from build123d import *

# Parameters (mm, degrees)
SKETCH_1_R          = 13.5
EXTRUDE_1_DEPTH     = 2
SKETCH_2_R          = 6.5
EXTRUDE_2_DEPTH     = 13
SKETCH_3_R          = 4
CUT_EXTRUDE_1_DEPTH = 15
SKETCH_4_R          = 1.5
CUT_EXTRUDE_2_DEPTH = 15


with BuildPart() as part:
    # 草图1 → 凸台-拉伸1 (new body)
    with BuildSketch(Plane.XY):
        Circle(SKETCH_1_R)
    extrude(amount=EXTRUDE_1_DEPTH)

    # 草图2 → 凸台-拉伸2 (add)
    with BuildSketch(Plane.XY.offset(2)):
        with Locations(Location((0, 0, 0), (0, 0, 180))):
            Circle(SKETCH_2_R)
    extrude(amount=EXTRUDE_2_DEPTH)

    # 草图3 → 切除-拉伸1 (cut)
    with BuildSketch(Plane.XY.offset(15)):
        Circle(SKETCH_3_R)
    extrude(amount=-CUT_EXTRUDE_1_DEPTH, mode=Mode.SUBTRACT)

    # 草图4 → 切除-拉伸2 (cut)
    with BuildSketch(Plane.XY.offset(2)):
        with Locations((-10.5, 0)):
            Circle(SKETCH_4_R)
        with Locations((-0.274707959, 10.5)):
            Circle(SKETCH_4_R)
        with Locations((10.5, 0)):
            Circle(SKETCH_4_R)
        with Locations((0, -10.5)):
            Circle(SKETCH_4_R)
    extrude(amount=-CUT_EXTRUDE_2_DEPTH, mode=Mode.SUBTRACT)


solid = part.part
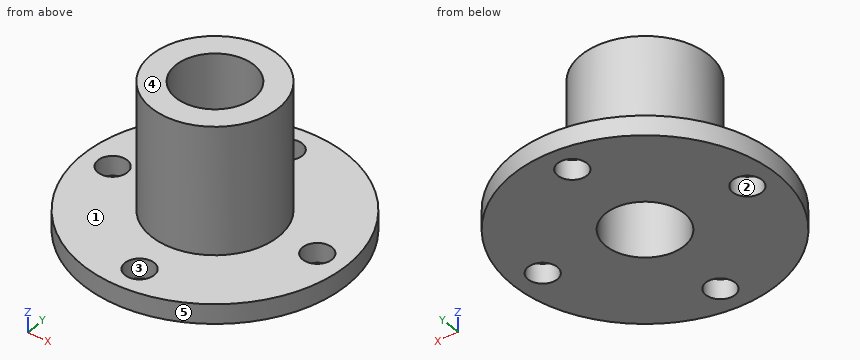
Could you check a few things on this model? Use its own coordinates, in mm. Face numbers are marked on the shaded views. A direction names the side the tool comes from. Round coordinates to 2 decimals unless told otherwise and drop trailing zeros. Loops run counter-clockwise (first coordinate to the right, second up) from the corner with the lowest first, then second, coordinate; pieces in that order, holes last. Notation, with made-up numbers: (-16.5, -31) - (-7.5, -31) arc R34 ccw to (-7.5, 3) - close; hole circle Ø3 at (70.25, 14). An arc over 180 degrees is marked (long way). Write item = value, one per line.
1) On a 3-axis mill with a long thin cutter (end or side, diameter ignored), from which of +Z, -Z, +X, -X, +Y, -Y can I reach the whole of each face in a straight line? I mean the marked faces 1 and 2. Say none if no direction works.
Computed:
face_1 = +Z
face_2 = +Z, -Z
2) Imagine slicing it at A-A (x = 0.5). Please give me the cut outline in (y, z).
Computed:
outline = (-13.49, 0) - (-11.91, 0) - (-11.91, 2) - (-13.49, 2) - close; (-9.09, 0) - (-3.97, 0) - (-3.97, 15) - (-6.48, 15) - (-6.48, 2) - (-9.09, 2) - close; (3.97, 0) - (9.22, 0) - (9.22, 2) - (6.48, 2) - (6.48, 15) - (3.97, 15) - close; (11.78, 0) - (13.49, 0) - (13.49, 2) - (11.78, 2) - close
3) Imagine slicing it at B-B (z = 1.5). Please give me the cut outline in (x, y), and give its area (3 significant figures).
Computed:
outline = circle Ø27 at (0, 0); hole circle Ø3 at (-10.5, 0); hole circle Ø8 at (0, 0); hole circle Ø3 at (-0.27, 10.5); hole circle Ø3 at (0, -10.5); hole circle Ø3 at (10.5, 0)
area = 494 mm2
4) Imagine slicing it at D-D (x = -2.75). Please give me the cut outline in (y, z).
Computed:
outline = (-13.22, 0) - (-2.9, 0) - (-2.9, 15) - (-5.89, 15) - (-5.89, 2) - (-13.22, 2) - close; (2.9, 0) - (13.22, 0) - (13.22, 2) - (5.89, 2) - (5.89, 15) - (2.9, 15) - close
5) I'm going to push flat-ended pins straight in: P1, Ø2.5, axis at x = -0.27, y = 10.5, coming from the -Z side; P2, Ø12, axis at x = 9, y = -10, coming from the +Z side; P3, Ø5, axis at y = -1, z = 4, coming from the +X side; P4, Ø2, axis at x = 3.5, z = 10.5, coming from the -Y side. Where does each tip first touch, or does it pass through?
Computed:
P1 = through
P2 = 2
P3 = 13.5
P4 = -6
6) If we mould it in two halves opening along Y, with no side actions, what happens to the marked faces 3, 4 and 5? For each: pulls with the +Y half, pulls with the -Y half, needs draft (parallel to the pull), parting line crosses it, or undercut.
Computed:
face_3 = undercut
face_4 = needs draft
face_5 = parting line crosses it
7) I need wall thicknesses on line 1 along Y through (x, z) = (0, 1.5); line 2 along Z through (x, y) = (9.25, -8); line 3 along X through (y, z) = (3.25, 7.75). Which ranges of each line are inside material? Lowest first, please. Write a range as from..to.
Computed:
line_1 = -13.5..-12, -9..-4, 4..9.03, 11.97..13.5
line_2 = 0..2
line_3 = -5.63..-2.33, 2.33..5.63
8) Imagine slicing it at C-C (y = -10). Please give me the cut outline in (x, z), and give its area (3 significant figures).
Computed:
outline = (-9.07, 0) - (-1.41, 0) - (-1.41, 2) - (-9.07, 2) - close; (1.41, 0) - (9.07, 0) - (9.07, 2) - (1.41, 2) - close
area = 30.6 mm2
